Geometry check sheet. Reference: drawing and pictorial views, mm from the part's lowest x, y, z. Round coordinates to 2 decimals unless told otherwise and drop trailing zeros. Order: outer loops, then holes, each group sorted by start corner. A loop starts at its lowest first (then second) coordinate and runs counter-clockwise, first axis right, second up. Notation, with made-up numbers: (-26.75, -29) -> (-20.75, -29) arc R17 ccw to (-20.75, -18) -> close; hole circle Ø9 at (60.25, 52). An arc over 180 degrees is marked (long way). Put each result on its own line as item: value.
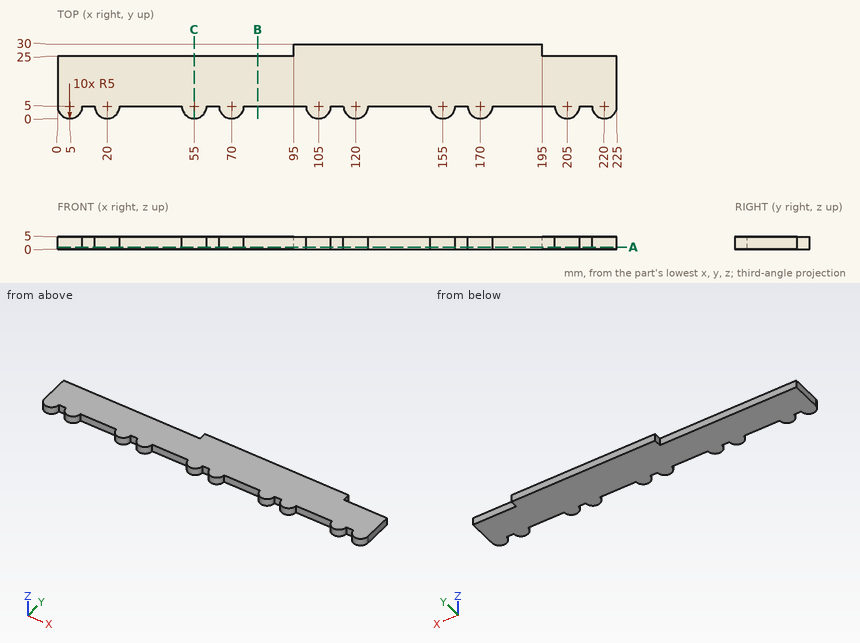
Item 1: Sectioned sample at A-A, the plane z = 0.8. Record the boundary of the cut face in (x, y), then the cut area to 3 significant figures.
Geometry check:
outline: (0, 5) arc R5 ccw to (10, 5) -> (15, 5) arc R5 ccw to (25, 5) -> (50, 5) arc R5 ccw to (60, 5) -> (65, 5) arc R5 ccw to (75, 5) -> (100, 5) arc R5 ccw to (110, 5) -> (115, 5) arc R5 ccw to (125, 5) -> (150, 5) arc R5 ccw to (160, 5) -> (165, 5) arc R5 ccw to (175, 5) -> (200, 5) arc R5 ccw to (210, 5) -> (215, 5) arc R5 ccw to (225, 5) -> (225, 25) -> (195, 25) -> (195, 30) -> (95, 30) -> (95, 25) -> (0, 25) -> close
area: 5,390 mm2
Item 2: Material ranges on line 1 along Y through (x, z) = (184, 4.7); line 2 along Y through (x, z) = (69.5, 3.5); line 3 along X through (y, z) = (26.5, 3.35), recorded low to high.
Geometry check:
line 1: 5 to 30
line 2: 0.03 to 25
line 3: 95 to 195
Item 3: Depth check by flat-ended pin: pin 1 Ø2.5 at (x, z) = (46, 3.5) entering from +Y; pin 2 Ø2.5 at (x, z) = (212, 2.5) entering from -Y; pin 3 Ø1.5 at (y, z) = (28, 1.5) entering from +X. Enter the tip coordinate at first touch or a pass-through.
Geometry check:
pin 1: y = 25
pin 2: y = 5
pin 3: x = 195
Item 4: Sectioned sample at C-C, the plane x = 55. Record the boundary of the cut face in (y, z), then the cut area to 3 significant figures.
Geometry check:
outline: (0, 0) -> (25, 0) -> (25, 5) -> (0, 5) -> close
area: 125 mm2
Item 5: Sectioned sample at B-B, the plane x = 80.5. Record the boundary of the cut face in (y, z).
Geometry check:
outline: (5, 0) -> (25, 0) -> (25, 5) -> (5, 5) -> close
